Solid Edge part; units mm, degrees
sketch "Sketch1" plane through (0, 0, 0) normal (0, 0, 1) x (1, 0, 0)
  line L0 (-76.1374, -248.5483) -> (423.8626, -248.5483)
  line L1 (423.8626, -248.5483) -> (423.8626, 51.4517)
  line L2 (423.8626, 51.4517) -> (-76.1374, 51.4517)
  line L3 (-76.1374, 51.4517) -> (-76.1374, -248.5483)
  dimension "D1" = 76.1374
  dimension "D2" = 423.8626
extrude "Protrusion1" add sketch "Sketch1" along normal blind 400
sketch "Sketch2" plane through (173.8626, -248.5483, 200) normal (0, -1, 0) x (1, 0, 0)
  line L0 (-144.6934, 217.7335) -> (290.7737, 30.9727)
  line L1 (290.7737, 30.9727) -> (282.4526, 244.5457)
  line L2 (282.4526, 244.5457) -> (-144.6934, 217.7335)
  line L3 (-218.6581, 177.053) -> (-212.1862, 117.8812)
  line L4 (-212.1862, 117.8812) -> (-72.5778, 117.8812)
  line L5 (-72.5778, 117.8812) -> (-85.5217, 177.053)
  line L6 (-85.5217, 177.053) -> (-218.6581, 177.053)
extrude "Cutout1" cut sketch "Sketch2" against normal through all
fillet "Round_3" radius 40 2 edges at (-76.1374, -98.5483, 400) (423.8626, -98.5483, 248.4595)
properties material "Aluminum, 6061-T6"
Read the model definition and answer for the solid it produces. Units are mm, in the model's axes. A direction names the side the tool comes from. Coordinates: 2 decimals unless noted, no trailing zeros. Write each loop counter-clockwise with the first axis right and the second up, starting at its lowest first coordinate (ties: lowest second). Pieces come first, ordered by that corner, then holes. Notation, with made-up numbers: (28, 86) - (77, 86) arc R25 cw to (77, 113) - close; hole circle Ø9 at (42, 22.25). An arc over 180 degrees is marked (long way). One line per question, with ' | ' between items.
Q1. Each of these flat-tipped pins is pushed along its axis until it touches: P1, Ø8, axis at x = 10, y = -139, coming from the -Z side; P2, Ø10, axis at x = 270.5, y = -156, coming from the +Z side; P3, Ø1, axis at y = 21, z = 311.5, coming from the +X side; P4, Ø2, axis at y = -152.5, z = 329.5, coming from the +X side. Where does it stop, or does it pass through?
Result set:
P1: z = 0 | P2: z = 316.38 | P3: x = 278.04 | P4: x = 237.23
Q2. For faces 1 (the flat face through (31, -101, 317.881)), 2 (the flat face through (170, -248.548, 153)), determine the directions among +Z, -Z, +X, -X, +Y, -Y from which every point of the face is accessible in a straight line to the end or side of a thin tool.
Result set:
face 1: +Y, -Y | face 2: +Z, -Z, +X, -X, -Y
Q3. Find section D-D, the plane x = 369. Write down the section's boundary in (y, z).
Result set:
outline: (-248.55, 0) - (51.45, 0) - (51.45, 271.99) - (-248.55, 271.99) - close
Q4. Find section B-B, the plane z = 329.5. Write down the section's boundary in (x, y), plus the area to 3 significant figures.
Result set:
outline: (-76.14, -248.55) - (-39.59, -248.55) - (-39.59, 51.45) - (-76.14, 51.45) - close; (98.74, -248.55) - (234.9, -248.55) - (234.9, 51.45) - (98.74, 51.45) - close | area: 51,800 mm^2
Q5. Consider L1, parallel to Z at x = 36.5, y = -148; L2, parallel to X at y = -67.5, z = 327; L3, parallel to X at y = -17.5, z = 374. Determine where each line is inside the solid, lowest interval first. Write a range as [from, to].
Result set:
L1: [0, 317.88], [377.05, 400] | L2: [-76.14, -39.32], [99.29, 240.73] | L3: [-73.61, -44.46], [89.01, 131.14]
Q6. Determine the mould class of faces 3 (the flat face through (94.903, -100.648, 347.053)), 4 (the flat face through (170, -96, 0)), 5 (the flat face through (423.863, -101, 109)) for opening direction X: +X half, -X half, draft (parallel to the pull), parting line (faces both ways), or undercut.
Result set:
face 3: undercut | face 4: draft | face 5: +X half
Q7. Find section C-C, the plane x = 81.5. Write down the section's boundary in (y, z).
Result set:
outline: (-248.55, 0) - (51.45, 0) - (51.45, 317.88) - (-248.55, 317.88) - close; (-248.55, 377.05) - (51.45, 377.05) - (51.45, 395.29) - (-248.55, 395.29) - close
Q8. Find section A-A, the plane y = 17. Write down the section's boundary in (x, z).
Result set:
outline: (-76.14, 0) - (423.86, 0) - (423.86, 222.09) arc R40 ccw to (399.63, 258.85) - (70.52, 400) - (-36.14, 400) arc R40 ccw to (-76.14, 360) - close; hole (-44.8, 377.05) - (-38.32, 317.88) - (101.28, 317.88) - (88.34, 377.05) - close
